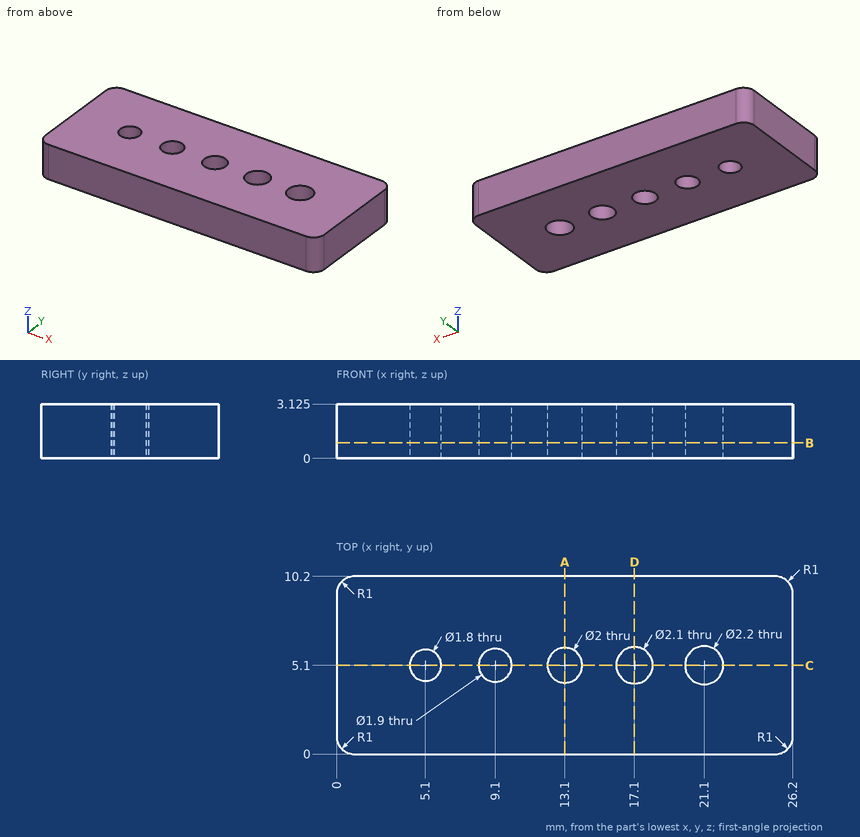
Geometry: see drawing. Coordinates: mm, zero at the bounding-box minimum. Coordinates: 2 decimals unless noted, no trailing zeros. Write each loop counter-clockwise with the first axis right and the second up, starting at its lowest first coordinate (ties: lowest second). Pieces come first, ordered by that corner, then holes. Notation, with made-up numbers: M 21,43 L 27,43 A23 ccw 27,58 Z; hole C 79,-13 d3. An arc over 180 degrees is marked long. Answer as a JSON object with one key per item and string values.
1. Cut plane B-B on z = 0.9. Output: boundary loops of the cut face in (x, y).
Evaluation:
{"outline": "M 0,1 A1 ccw 1,0 L 25.2,0 A1 ccw 26.2,1 L 26.2,9.2 A1 ccw 25.2,10.2 L 1,10.2 A1 ccw 0,9.2 Z; hole C 5.1,5.1 d1.8; hole C 9.1,5.1 d1.9; hole C 13.1,5.1 d2; hole C 17.1,5.1 d2.1; hole C 21.1,5.1 d2.2"}
2. Ray query, L1, parallel to Y at x = 13.1, z = 1.75; L2, parallel to Y at x = 5.1, z = 1.2; L3, parallel to X at y = 5, z = 1.3. Return the intervals inside material, ascending.
Evaluation:
{"L1": "0 to 4.1, 6.1 to 10.2", "L2": "0 to 4.2, 6 to 10.2", "L3": "0 to 4.21, 5.99 to 8.16, 10.04 to 12.11, 14.09 to 16.05, 18.15 to 20, 22.2 to 26.2"}
3. Cut plane D-D on x = 17.1. Output: boundary loops of the cut face in (y, z) (3 decimals), plus the area to 3 significant figures.
Evaluation:
{"outline": "M 0,0 L 4.05,0 L 4.05,3.125 L 0,3.125 Z; M 6.15,0 L 10.2,0 L 10.2,3.125 L 6.15,3.125 Z", "area": "25.3 mm^2"}
4. Cut plane C-C on y = 5.1. Output: boundary loops of the cut face in (x, z) (3 decimals).
Evaluation:
{"outline": "M 0,0 L 4.2,0 L 4.2,3.125 L 0,3.125 Z; M 6,0 L 8.15,0 L 8.15,3.125 L 6,3.125 Z; M 10.05,0 L 12.1,0 L 12.1,3.125 L 10.05,3.125 Z; M 14.1,0 L 16.05,0 L 16.05,3.125 L 14.1,3.125 Z; M 18.15,0 L 20,0 L 20,3.125 L 18.15,3.125 Z; M 22.2,0 L 26.2,0 L 26.2,3.125 L 22.2,3.125 Z"}
5. Cut plane A-A on x = 13.1. Output: boundary loops of the cut face in (y, z) (3 decimals), plus the area to 3 significant figures.
Evaluation:
{"outline": "M 0,0 L 4.1,0 L 4.1,3.125 L 0,3.125 Z; M 6.1,0 L 10.2,0 L 10.2,3.125 L 6.1,3.125 Z", "area": "25.6 mm^2"}
